```python
from build123d import *

# Parameters (mm, degrees)
CUT_EXTRUDE_START    = -53.5
SKETCH_2_OUTSIDE_W   = 231.472
SKETCH_2_OUTSIDE_H   = 231.472
CUT_EXTRUDE_1_DEPTH  = 35
CUT_EXTRUDE_START_2  = 53.5
SKETCH_2_2_OUTSIDE_W = 231.472
SKETCH_2_2_OUTSIDE_H = 231.472
CUT_EXTRUDE_2_DEPTH  = 35
SKETCH_3_R           = 53
CUT_EXTRUDE_3_DEPTH  = 42


with BuildPart() as part:
    # Эскиз1 → Повернуть1 (revolve)
    with BuildSketch(Plane.XY):
        Polygon((32.5, 85), (37.5, 85), (37.5, 80), (45.5, 53), (45.5, 11), (48.5, 11), (48.5, 8), (87.5, 8), (87.5, 0), (-87.5, 0), (-87.5, 8), (-48.5, 8), (-48.5, 11), (-45.5, 11), (-45.5, 53), (-37.5, 80), (-37.5, 85), (-32.5, 85), (-32.5, 78), (32.5, 78), align=None)
    revolve(axis=Axis((-1100.903674864, 0, 0), (1, 0, 0)))

    # Эскиз2 outside → Вырез-Вытянуть1 (cut, through all)
    with BuildSketch(Plane(origin=(0, 0, 0), x_dir=(0, 0, -1), z_dir=(1, 0, 0)).offset(CUT_EXTRUDE_START)):
        Rectangle(SKETCH_2_OUTSIDE_W, SKETCH_2_OUTSIDE_H)
        with BuildLine():
            Line((-6, 5.291502622), (-6, -5.291502622))
            ThreePointArc((-6, -5.291502622), (0, -8), (6, -5.291502622))
            Line((6, -5.291502622), (6, 5.291502622))
            ThreePointArc((6, 5.291502622), (0, 8), (-6, 5.291502622))
        make_face(mode=Mode.SUBTRACT)
    extrude(amount=-CUT_EXTRUDE_1_DEPTH, mode=Mode.SUBTRACT)

    # Эскиз2<2> outside → Вырез-Вытянуть2 (cut, through all)
    with BuildSketch(Plane(origin=(0, 0, 0), x_dir=(0, 0, -1), z_dir=(1, 0, 0)).offset(CUT_EXTRUDE_START_2)):
        Rectangle(SKETCH_2_2_OUTSIDE_W, SKETCH_2_2_OUTSIDE_H)
        with BuildLine():
            Line((-6, 5.291502622), (-6, -5.291502622))
            ThreePointArc((-6, -5.291502622), (0, -8), (6, -5.291502622))
            Line((6, -5.291502622), (6, 5.291502622))
            ThreePointArc((6, 5.291502622), (0, 8), (-6, 5.291502622))
        make_face(mode=Mode.SUBTRACT)
    extrude(amount=CUT_EXTRUDE_2_DEPTH, mode=Mode.SUBTRACT)

    # Эскиз3 → Вырез-Вытянуть3 (cut)
    with BuildSketch(Plane(origin=(87.5, 0, 0), x_dir=(0, 0, -1), z_dir=(1, 0, 0))):
        Circle(SKETCH_3_R)
    extrude(amount=-CUT_EXTRUDE_3_DEPTH, mode=Mode.SUBTRACT)


solid = part.part
```
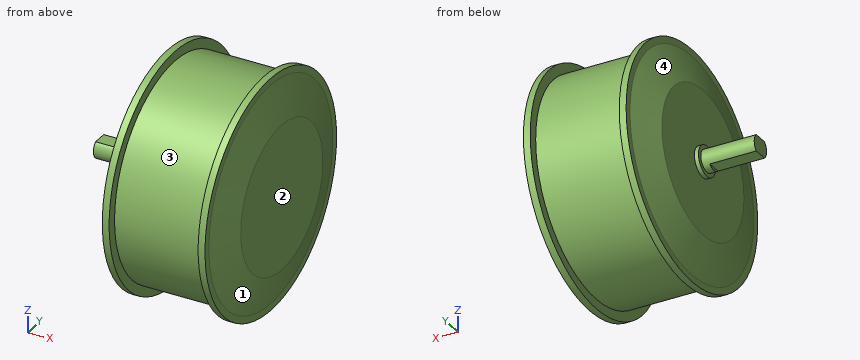
Build history of the part. All positions in model axes, mm. Face numbers are marked on the shaded views. A direction names the side the tool comes from. Give positions to 0.01 mm unless a question says otherwise; leave off trailing zeros. Loops run counter-clockwise (first coordinate to the right, second up) from the corner with the lowest first, then second, coordinate; pieces in that order, holes last. Notation, with made-up numbers: (21, -12.5) -> (76, -12.5) arc R23 cw to (76, 8.5) -> close; hole circle Ø4 at (19.5, 79.25). An arc over 180 degrees is marked (long way). One line per question, with ' | ' between items. Start each with the question number.
1) Cut at D-D (x = -67). Give the cut face in (y, z), plus the area to 3 significant figures.
2) 3-axis set-ups, long thin cutter, end or side, ignore diameter. For the marked faces 3 and 4: which of +Z, -Z, +X, -X, +Y, -Y reach the whole face in a straight line?
3) Pin check, flat tips, straight feed: pin 1 (8 mm diameter, centred on y = 38.5, z = 57.5, fed in from +X); pin 2 (11.5 mm diameter, centred on x = -65, y = 0, fed in from +Z); pin 3 (0.6 mm diameter, centred on y = -2, z = 7, fed in from -X). Stop position of each tip, or through.
4) Cut at A-A (z = 0). Give the cut face in (x, y).
5) Cut at C-C (x = 12). Give the cut face in (y, z), plus the area to 3 significant figures.
6) Probe L1, parallel to X at y = -63, z = -53.5; L2, parallel to X at y = -0.5, z = 30.5; L3, parallel to Y at x = -19, z = 66. List the from-to ranges inside material, lowest first.
7) Two-plate mould, pull along Z, no slides. Class the marked faces 1 and 2: released by +Z, released by -Z, zero draft, split by the parting line, or undercut.
Return value:
1) outline: (-5.29, -6) -> (5.29, -6) arc R8 ccw to (5.29, 6) -> (-5.29, 6) arc R8 ccw to start | area: 172 mm^2
2) face 3: none | face 4: -X
3) pin 1: x = 41.89 | pin 2: z = 6 | pin 3: x = -53.5
4) outline: (-87.5, -8) -> (-48.5, -8) -> (-48.5, -11) -> (-45.5, -11) -> (-45.5, -53) -> (-37.5, -80) -> (-37.5, -85) -> (-32.5, -85) -> (-32.5, -78) -> (32.5, -78) -> (32.5, -85) -> (37.5, -85) -> (37.5, -80) -> (45.5, -53) -> (45.5, 53) -> (37.5, 80) -> (37.5, 85) -> (32.5, 85) -> (32.5, 78) -> (-32.5, 78) -> (-32.5, 85) -> (-37.5, 85) -> (-37.5, 80) -> (-45.5, 53) -> (-45.5, 11) -> (-48.5, 11) -> (-48.5, 8) -> (-87.5, 8) -> close
5) outline: circle Ø156 at (0, 0) | area: 19,100 mm^2
6) L1: -37.5 to -32.5, 32.5 to 37.5 | L2: -45.5 to 45.5 | L3: -41.57 to 41.57
7) face 1: split by the parting line | face 2: zero draft
